from build123d import *

# Parameters (mm, degrees)
F0_R          = 8.5
F1_DEPTH      = 101
F1_DEPTH_BACK = 101
F2_SIZE       = 1.5
F4_W          = 8.5
F4_H          = 22
F5_DEPTH      = 1.5


with BuildPart() as f1:
    # F0 (on Front) → F1 (new body, two sides)
    with BuildSketch(Plane.XZ) as f1_sk:
        Circle(F0_R)
    extrude(amount=F1_DEPTH)
    extrude(f1_sk.sketch, amount=-F1_DEPTH_BACK)

    # F2
    f2_edges = [f1.edges().sort_by_distance(p)[0] for p in [
        (-8.5, -101, 0),
        (-8.5, 101, 0),
    ]]
    chamfer(f2_edges, length=F2_SIZE)

    # F4 (on offset) → F5 (cut)
    with BuildSketch(Plane.XY.offset(8.5)):
        with Locations((0, -90)):
            Rectangle(F4_W, F4_H)
    extrude(amount=-F5_DEPTH, mode=Mode.SUBTRACT)


solid = f1.part
Verification items for the finished model (mm, model axes). Coordinates: 2 decimals unless noted, no trailing zeros. Loops run counter-clockwise (first coordinate to the right, second up) from the corner with the lowest first, then second, coordinate; pieces in that order, holes last. Notation, with made-up numbers: (61, 11.5) -> (75, 11.5) arc R32 cw to (75, 42.5) -> close; hole circle Ø4 at (83, 72.25). An arc over 180 degrees is marked (long way). Write each question's results on one line, items separated by ' | '.
Item 1: Section check A-A, the plane y = -24. Enter the section's corners in (x, z), plus the area to 3 significant figures.
Found:
outline: circle Ø17 at (0, 0) | area: 227 mm2
Item 2: Mould release check, pull along X, two halves, no side actions. Record for faces 1 (the face through (0, 101, 0)), 2 (the face through (-1.84, -1.39, -8.3)), 3 (the face through (0, -90, 7)): +X half, -X half, draft (parallel to the pull), parting line (faces both ways), or undercut.
Found:
face 1: draft | face 2: parting line | face 3: undercut
Item 3: Gauge pin test, flat ends, axial feed: pin 1 (3 mm diameter, centred on y = -58.5, z = 6, fed in from -X); pin 2 (2 mm diameter, centred on x = 3, y = -0.5, fed in from -Z); pin 3 (9.5 mm diameter, centred on x = 0, y = -94.5, fed in from +Z). Record the tip position at first contact, or that the pin passes through.
Found:
pin 1: stops at x = -7.21 | pin 2: stops at z = -8.26 | pin 3: stops at z = 7.36
Item 4: Material ranges on L1, parallel to Y at x = -7, z = -4.75; L2, parallel to X at y = -90, z = -0.25; L3, parallel to Z at x = 2.25, y = 3, recorded low to high.
Found:
L1: y = -99.54 to 99.54 | L2: x = -8.5 to 8.5 | L3: z = -8.2 to 8.2
